Part model, mm, in its own coordinate system. A direction names the side the tool comes from. Round coordinates to 2 decimals unless told otherwise and drop trailing zeros. Loops run counter-clockwise (first coordinate to the right, second up) from the corner with the lowest first, then second, coordinate; pieces in that order, holes last. Notation, with made-up numbers: (47.5, 31) -> (74.5, 31) arc R23 cw to (74.5, 45) -> close; hole circle Ø3 at (-4.75, 84.25). An arc over 180 degrees is marked (long way). Use a Markdown table: item, result. Add a question column.
Item 1: Which spindle directions (+Z, -Z, +X, -X, +Y, -Y) get a long thin tool onto all of the face, cutting with end or side? Do faces 4 (the face through (1, 14, 0)), 5 (the face through (1, 20.142, -22)). Say none if no direction does.
Item 2: Probe line 1 (Z direction, x = 1.4, y = 21.25); line 2 (Y direction, x = 0.65, z = -23); line 3 (Y direction, x = 0.4, z = -9). List the from-to ranges inside material, lowest first. Write a range as [from, to].
Item 3: Cut at B-B, the plane z = -3.81. List the corners of the cut face in (x, y), plus the area to 3 significant figures.
Item 4: Two-plate mould, pull along Y, no slides. Class faces 1 (the face through (1, 27.94, -14)), 2 (the face through (1.727, 15, -14)), 3 (the face through (1, 21.869, -22)): pulls with the +Y half, pulls with the -Y half, needs draft (parallel to the pull), parting line crosses it, or undercut.
Item 5: Cut at C-C, the plane z = -11. List the corners of the cut face in (x, y), plus the area to 3 significant figures.
Item 6: Cut at D-D, the plane x = 0.55. State how many separate pieces and enclosed holes the cut face has, plus the area to 3 significant figures.
Item 7: Cut at A-A, the plane y = 24.5. List the corners of the cut face in (x, z), plus the area to 3 significant figures.
```python
from build123d import *

# Parameters (mm, degrees)
SKETCH1_W           = 27.94
SKETCH1_H           = 27.94
SKETCH1_W_2         = 6.35
SKETCH1_H_2         = 6.35
SKETCH1_W_3         = 1.7272
SKETCH1_H_3         = 2.032
BOSS_EXTRUDE1_DEPTH = 1.7272
SKETCH4_R           = 4.572
SKETCH4_R_2         = 2.794
CUT_EXTRUDE4_DEPTH  = 1.7272
SKETCH8_W           = 1.7272
SKETCH8_H           = 2.032
CUT_EXTRUDE5_DEPTH  = 1.7272
SKETCH9_W           = 1.7272
SKETCH9_H           = 2.032
CUT_EXTRUDE6_DEPTH  = 1.7272
SKETCH10_W          = 27.94
SKETCH10_H          = 1.27
CUT_EXTRUDE7_DEPTH  = 1.7272


with BuildPart() as part:
    # Sketch1 → Boss-Extrude1 (new body)
    with BuildSketch(Plane(origin=(0, 0, 0), x_dir=(0, 0, -1), z_dir=(1, 0, 0))):
        with Locations((13.97, 13.97)):
            Rectangle(SKETCH1_W, SKETCH1_H)
        with Locations((8.89, 7.747)):
            Rectangle(SKETCH1_W_2, SKETCH1_H_2, mode=Mode.SUBTRACT)
        with Locations((26.5684, 4.191)):
            Rectangle(SKETCH1_W_3, SKETCH1_H_3, mode=Mode.SUBTRACT)
        with Locations((26.5684, 24.511)):
            Rectangle(SKETCH1_W_3, SKETCH1_H_3, mode=Mode.SUBTRACT)
    extrude(amount=BOSS_EXTRUDE1_DEPTH)

    # Sketch4 → Cut-Extrude4 (cut)
    with BuildSketch(Plane(origin=(1.7272, 0, 0), x_dir=(0, 0, -1), z_dir=(1, 0, 0))):
        with BuildLine():
            ThreePointArc((9.569657679, 10.922), (12.354864998, 12.460266118), (13.462, 15.4432))
            ThreePointArc((13.462, 15.4432), (10.193220511, 19.825528183), (5.06095, 17.941511449))
            ThreePointArc((5.06095, 17.941511449), (6.18714012, 16.911410084), (6.604, 15.4432))
            ThreePointArc((6.604, 15.4432), (6.18714012, 13.974989916), (5.06095, 12.944888551))
            ThreePointArc((5.06095, 12.944888551), (6.41914372, 11.596376213), (8.210342321, 10.922))
            Line((8.210342321, 10.922), (9.569657679, 10.922))
        make_face()
        with Locations((8.89, 15.4432)):
            Circle(SKETCH4_R)
        with Locations((3.81, 15.4432)):
            Circle(SKETCH4_R_2)
    extrude(amount=-CUT_EXTRUDE4_DEPTH, mode=Mode.SUBTRACT)

    # Sketch8 → Cut-Extrude5 (cut)
    with BuildSketch(Plane(origin=(0, 20.1422, 3.5052), x_dir=(0, -1, 0), z_dir=(1, 0, 0))):
        with Locations((-0.8636, 25.7048)):
            Rectangle(SKETCH8_W, SKETCH8_H)
        with Locations((-0.8636, 5.3848)):
            Rectangle(SKETCH8_W, SKETCH8_H)
    extrude(amount=CUT_EXTRUDE5_DEPTH, mode=Mode.SUBTRACT)

    # Sketch9 → Cut-Extrude6 (cut)
    with BuildSketch(Plane(origin=(0, 2.3622, 3.5052), x_dir=(0, -1, 0), z_dir=(1, 0, 0))):
        with Locations((-0.8636, 25.7048)):
            Rectangle(SKETCH9_W, SKETCH9_H)
        with Locations((-0.8636, 5.3848)):
            Rectangle(SKETCH9_W, SKETCH9_H)
    extrude(amount=CUT_EXTRUDE6_DEPTH, mode=Mode.SUBTRACT)

    # Sketch10 → Cut-Extrude7 (cut)
    with BuildSketch(Plane(origin=(1.7272, 0, 0), x_dir=(0, 0, -1), z_dir=(1, 0, 0))):
        with Locations((13.97, 0.635)):
            Rectangle(SKETCH10_W, SKETCH10_H)
    extrude(amount=-CUT_EXTRUDE7_DEPTH, mode=Mode.SUBTRACT)


solid = part.part
```
A:
| question | item | result |
|---|---|---|
| 1 | face 4 | +Z, +X, -X, +Y, -Y |
| 1 | face 5 | +X, -X |
| 2 | line 1 | z = [-27.94, -23.22], [-21.18, -2.9], [-0.86, 0] |
| 2 | line 2 | y = [1.27, 2.36], [4.09, 20.14], [21.87, 27.94] |
| 2 | line 3 | y = [1.27, 4.57], [20.01, 27.94] |
| 3 | outline | (0, 1.27) -> (1.73, 1.27) -> (1.73, 12.65) -> (0, 12.65) -> close; (0, 18.24) -> (1.73, 18.24) -> (1.73, 27.94) -> (0, 27.94) -> close |
| 3 | area | 36.4 mm^2 |
| 4 | face 1 | pulls with the +Y half |
| 4 | face 2 | needs draft |
| 4 | face 3 | undercut |
| 5 | outline | (0, 1.27) -> (1.73, 1.27) -> (1.73, 4.57) -> (0, 4.57) -> close; (0, 10.92) -> (1.73, 10.92) -> (1.73, 11.39) -> (0, 11.39) -> close; (0, 19.5) -> (1.73, 19.5) -> (1.73, 27.94) -> (0, 27.94) -> close |
| 5 | area | 21.1 mm^2 |
| 6 | separate pieces | 1 |
| 6 | enclosed holes | 7 |
| 6 | area | 602 mm^2 |
| 7 | outline | (0, -27.94) -> (1.73, -27.94) -> (1.73, -27.43) -> (0, -27.43) -> close; (0, -25.7) -> (1.73, -25.7) -> (1.73, 0) -> (0, 0) -> close |
| 7 | area | 45.3 mm^2 |
